from build123d import *

# Parameters (mm, degrees)
SKETCH1_R           = 2.25
SKETCH1_R_2         = 2.75
BOSS_EXTRUDE1_DEPTH = 2.5
CHAMFER1_SIZE       = 2


with BuildPart() as part:
    # Sketch1 → Boss-Extrude1 (new body, symmetric)
    with BuildSketch(Plane.XY):
        with BuildLine():
            Line((-117.5, -12.8), (137.5, -12.8))
            ThreePointArc((137.5, -12.8), (147.382444583, -4.328819498), (140.521694793, 6.732542189))
            Line((140.521694793, 6.732542189), (107.5, 17.2))
            Line((107.5, 17.2), (-107.5, 17.2))
            Line((-107.5, 17.2), (-123.5, 5.2))
            ThreePointArc((-123.5, 5.2), (-126.986832981, -5.96227766), (-117.5, -12.8))
        make_face()
        with Locations((75, 0)):
            Circle(SKETCH1_R, mode=Mode.SUBTRACT)
        with Locations((-75, 0)):
            Circle(SKETCH1_R, mode=Mode.SUBTRACT)
        with Locations((-117.5, -2.8)):
            Circle(SKETCH1_R_2, mode=Mode.SUBTRACT)
        with Locations((117.5, -2.8)):
            Circle(SKETCH1_R_2, mode=Mode.SUBTRACT)
        with Locations((137.5, -2.8)):
            Circle(SKETCH1_R_2, mode=Mode.SUBTRACT)
    extrude(amount=BOSS_EXTRUDE1_DEPTH, both=True)

    # Chamfer1
    chamfer1_edges = [part.edges().sort_by_distance(p)[0] for p in [
        (-77.25, 0, 2.5),
        (72.75, 0, 2.5),
    ]]
    chamfer(chamfer1_edges, length=CHAMFER1_SIZE)


solid = part.part
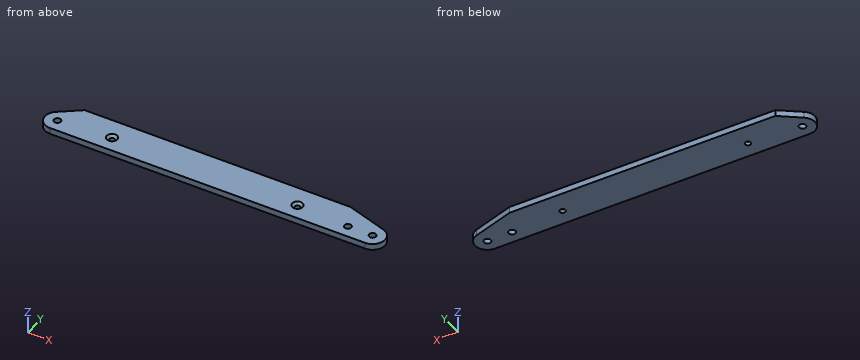
Work out the finished part from the listing and answer in its coordinate system (mm). Give positions to 0.01 mm unless a question says otherwise; leave off trailing zeros. Order: outer loops, then holes, each group sorted by start corner. A loop starts at its lowest first (then second) coordinate and runs counter-clockwise, first axis right, second up. Notation, with made-up numbers: (29, -19) -> (39, -19) arc R13 ccw to (39, -3) -> close; hole circle Ø11 at (-4, 57). An arc over 180 degrees is marked (long way). Answer as a JSON object with one key per item and string values. Group by question number.
1. Section A-A on z = -1.7 is taken. Determine the outline of the cut face in (x, y).
2. Section C-C on y = 13.5 is taken. Determine the outline of the cut face in (x, z), plus the area to 3 significant figures.
3. Section B-B on x = 117.5 is taken. Determine the outline of the cut face in (y, z), plus the area to 3 significant figures.
4. Consider line 1 along Y through (x, z) = (75, -1); line 2 along X through (y, z) = (2, -1.45); line 3 along X through (y, z) = (-4, 2). Determine where each line is inside the solid, lowest interval first. Write a range as [from, to].
5. Flat-ended cylindrical pins translate along their axes: pin 1 Ø3.5 at (x, y) = (-75, 0) entering from -Z; pin 2 Ø9 at (x, y) = (137.5, -2.8) entering from -Z; pin 3 Ø6 at (x, y) = (75, 0) entering from +Z. Find the tip coordinate at first contact, or state that the pin passes through.
Result sheet:
{
 "1": {"outline": "(-123.5, 5.2) arc R10 ccw to (-117.5, -12.8) -> (137.5, -12.8) arc R10 ccw to (140.52, 6.73) -> (107.5, 17.2) -> (-107.5, 17.2) -> close; hole circle Ø5.5 at (-117.5, -2.8); hole circle Ø4.5 at (-75, 0); hole circle Ø4.5 at (75, 0); hole circle Ø5.5 at (117.5, -2.8); hole circle Ø5.5 at (137.5, -2.8)"},
 "2": {"outline": "(-112.43, -2.5) -> (119.17, -2.5) -> (119.17, 2.5) -> (-112.43, 2.5) -> close", "area": "1,160 mm^2"},
 "3": {"outline": "(-12.8, -2.5) -> (-5.55, -2.5) -> (-5.55, 2.5) -> (-12.8, 2.5) -> close; (-0.05, -2.5) -> (14.03, -2.5) -> (14.03, 2.5) -> (-0.05, 2.5) -> close", "area": "107 mm^2"},
 "4": {"line 1": "y = [-12.8, -2.25], [2.25, 17.2]", "line 2": "x = [-126.27, -76.03], [-73.97, 73.97], [76.03, 146.27]", "line 3": "x = [-127.43, -119.97], [-115.03, 115.03], [119.97, 135.03], [139.97, 147.43]"},
 "5": {"pin 1": "passes through", "pin 2": "stops at z = -2.5", "pin 3": "stops at z = 1.25"}
}
